CAD build for the part. Positions are in the model's coordinates, mm. A direction names the side the tool comes from. Coordinates: 2 decimals unless noted, no trailing zeros. Order: outer loops, then holes, each group sorted by start corner. A loop starts at its lowest first (then second) coordinate and runs counter-clockwise, first axis right, second up. Notation, with made-up numbers: (52, 51.5) - (61, 51.5) arc R31 cw to (61, 89.5) - close; hole circle Ø6 at (70, 83). An arc over 180 degrees is marked (long way). Write each question's results on one line, items separated by ' | '. Start each with the question number.
Q1. Band-saw the part on D-D, the plane z = 24.4. Write the cut outline in (x, y), then the cut area to 3 significant figures.
Q2. Band-saw the part on B-B, the plane z = -5.5. Write the cut outline in (x, y), then the cut area to 3 significant figures.
Q3. Band-saw the part on C-C, the plane y = 12. Write the cut outline in (x, z).
Q4. Band-saw the part on A-A, the plane x = 5.2. Write the cut outline in (y, z).
Q5. Pin check, flat tips, straight feed: P1, Ø1, axis at x = -9.5, y = 10, coming from the -Z side; P2, Ø3.5, axis at x = 7, y = 16.5, coming from the +Z side; P3, Ø3.5, axis at x = 5.2, z = 23.8, coming from the -Y side. Stop position of each tip, or through.
Q6. Wall check: probe 1 along Z at (x, y) = (5.2, 26.4); probe 2 along X at (y, z) = (26.3, -23.8); probe 3 along Z at (x, y) = (-7, 20.5). Give the ranges that are in metal, low to high.
Q7. Which spindle directions (+Z, -Z, +X, -X, +Y, -Y) get a long thin tool onto all of the face, cutting with end or side? Do faces 4 (the flat face through (-3, 26, -22.5)), 5 (the flat face through (-10.1, 13, -26)), 6 (the flat face through (1, 24.9, 24)). Say none if no direction does.
Q8. Pull direction Z, two halves, no side cores. Call faces 1 (the flat face through (-11, 26.9, 0)), 2 (the flat face through (-11, 18, 27.5)), 3 (the flat face through (0, 14, 20.1)): released by +Z, released by -Z, zero draft, split by the parting line, or undercut.
```python
from build123d import *

# Parameters (mm, degrees)
SKETCH2_W           = 75
SKETCH2_H           = 8
SKETCH2_R           = 1.6
BOSS_EXTRUDE1_DEPTH = 2
SKETCH3_W           = 25
SKETCH3_H           = 18.5
BOSS_EXTRUDE2_DEPTH = 2
SKETCH4_W           = 25
SKETCH4_H           = 2
BOSS_EXTRUDE3_DEPTH = 18.5
SKETCH5_W           = 10.2
SKETCH5_H           = 40.2
CUT_EXTRUDE1_DEPTH  = 18.5
SKETCH6_W           = 10.2
SKETCH6_H           = 40.2
BOSS_EXTRUDE4_DEPTH = 24.9
SKETCH8_W           = 25
SKETCH8_H           = 7
BOSS_EXTRUDE5_DEPTH = 2
SKETCH9_R           = 1.6
CUT_EXTRUDE2_DEPTH  = 2
SKETCH10_W          = 20.2
SKETCH10_H          = 40.2
CUT_EXTRUDE3_DEPTH  = 77
SKETCH11_W          = 7
SKETCH11_H          = 2.4
CUT_EXTRUDE4_DEPTH  = 77
SKETCH12_W          = 2.4
SKETCH12_H          = 7
BOSS_EXTRUDE6_DEPTH = 24.9
SKETCH13_W          = 4
SKETCH13_H          = 4
CUT_EXTRUDE5_DEPTH  = 77
SKETCH14_W          = 25
SKETCH14_H          = 8
SKETCH14_R          = 1.6
BOSS_EXTRUDE7_DEPTH = 2
CUT_EXTRUDE6_DEPTH  = 2
CHAMFER1_SIZE       = 10
CUT_EXTRUDE7_DEPTH  = 1.2
SKETCH17_W          = 20.2
SKETCH17_H          = 22.9
CUT_EXTRUDE8_DEPTH  = 1.2
CUT_EXTRUDE9_DEPTH  = 2
CUT_EXTRUDE10_DEPTH = 2
SKETCH20_W          = 25
SKETCH20_H          = 8
CUT_EXTRUDE11_DEPTH = 156
SKETCH21_W          = 6.2
SKETCH21_H          = 22.9
CUT_EXTRUDE12_DEPTH = 55
SKETCH22_R          = 1.6
CUT_EXTRUDE13_DEPTH = 55


with BuildPart() as part:
    # Sketch2 → Boss-Extrude1 (new body)
    with BuildSketch(Plane(origin=(0, 0, 0), x_dir=(1, 0, 0), z_dir=(0, 1, 0))):
        Rectangle(SKETCH2_W, SKETCH2_H)
        with Locations((-31.75, 0)):
            Circle(SKETCH2_R, mode=Mode.SUBTRACT)
        with Locations((31.75, 0)):
            Circle(SKETCH2_R, mode=Mode.SUBTRACT)
    extrude(amount=BOSS_EXTRUDE1_DEPTH)

    # Sketch3 → Boss-Extrude2 (add)
    with BuildSketch(Plane(origin=(0, 2, 0), x_dir=(1, 0, 0), z_dir=(0, 1, 0))):
        with Locations((0, -13.25)):
            Rectangle(SKETCH3_W, SKETCH3_H)
    extrude(amount=-BOSS_EXTRUDE2_DEPTH)

    # Sketch4 → Boss-Extrude3 (add)
    with BuildSketch(Plane(origin=(0, 0, -4), x_dir=(-1, 0, 0), z_dir=(0, 0, -1))):
        with Locations((0, 1)):
            Rectangle(SKETCH4_W, SKETCH4_H)
    extrude(amount=BOSS_EXTRUDE3_DEPTH)

    # Sketch5 → Cut-Extrude1 (cut)
    with BuildSketch(Plane(origin=(0, 2, 0), x_dir=(1, 0, 0), z_dir=(0, 1, 0))):
        Rectangle(SKETCH5_W, SKETCH5_H)
    extrude(amount=-CUT_EXTRUDE1_DEPTH, mode=Mode.SUBTRACT)

    # Sketch6 → Boss-Extrude4 (add)
    with BuildSketch(Plane(origin=(0, 2, 0), x_dir=(1, 0, 0), z_dir=(0, 1, 0))):
        Polygon((-12.5, 4), (-12.5, -4), (-12.5, -22.5), (12.5, -22.5), (12.5, -4), (12.5, 4), (12.5, 22.5), (-12.5, 22.5), align=None)
        Rectangle(SKETCH6_W, SKETCH6_H, mode=Mode.SUBTRACT)
    extrude(amount=BOSS_EXTRUDE4_DEPTH)

    # Sketch8 → Boss-Extrude5 (add)
    with BuildSketch(Plane(origin=(0, 26.9, 0), x_dir=(1, 0, 0), z_dir=(0, 1, 0))):
        with Locations((0, 26)):
            Rectangle(SKETCH8_W, SKETCH8_H)
        with Locations((0, -26)):
            Rectangle(SKETCH8_W, SKETCH8_H)
    extrude(amount=-BOSS_EXTRUDE5_DEPTH)

    # Sketch9 → Cut-Extrude2 (cut)
    with BuildSketch(Plane.XZ.offset(-24.9)):
        with Locations((5.2, 23.8)):
            Circle(SKETCH9_R)
        with Locations((-5.2, 23.8)):
            Circle(SKETCH9_R)
        with Locations((-5.2, -23.8)):
            Circle(SKETCH9_R)
        with Locations((5.2, -23.8)):
            Circle(SKETCH9_R)
    extrude(amount=-CUT_EXTRUDE2_DEPTH, mode=Mode.SUBTRACT)

    # Sketch10 → Cut-Extrude3 (cut)
    with BuildSketch(Plane.XZ):
        Rectangle(SKETCH10_W, SKETCH10_H)
    extrude(amount=-CUT_EXTRUDE3_DEPTH, mode=Mode.SUBTRACT)

    # Sketch11 → Cut-Extrude4 (cut)
    with BuildSketch(Plane.XZ):
        with Locations((0, -21.3)):
            Rectangle(SKETCH11_W, SKETCH11_H)
    extrude(amount=-CUT_EXTRUDE4_DEPTH, mode=Mode.SUBTRACT)

    # Sketch12 → Boss-Extrude6 (add)
    with BuildSketch(Plane.XZ):
        with Locations((-11.3, 26)):
            Rectangle(SKETCH12_W, SKETCH12_H)
        with Locations((-11.3, -26)):
            Rectangle(SKETCH12_W, SKETCH12_H)
        with Locations((11.3, 26)):
            Rectangle(SKETCH12_W, SKETCH12_H)
        with Locations((11.3, -26)):
            Rectangle(SKETCH12_W, SKETCH12_H)
    extrude(amount=-BOSS_EXTRUDE6_DEPTH)

    # Sketch13 → Cut-Extrude5 (cut)
    with BuildSketch(Plane(origin=(0, 26.9, 0), x_dir=(1, 0, 0), z_dir=(0, 1, 0))):
        with Locations((0, 22.5)):
            Rectangle(SKETCH13_W, SKETCH13_H)
    extrude(amount=-CUT_EXTRUDE5_DEPTH, mode=Mode.SUBTRACT)

    # Sketch14 → Boss-Extrude7 (add)
    with BuildSketch(Plane(origin=(0, 2, 0), x_dir=(1, 0, 0), z_dir=(0, 1, 0))):
        with Locations((-25, 0)):
            Rectangle(SKETCH14_W, SKETCH14_H)
        with Locations((-31.75, 0)):
            Circle(SKETCH14_R, mode=Mode.SUBTRACT)
        with Locations((25, 0)):
            Rectangle(SKETCH14_W, SKETCH14_H)
        with Locations((31.75, 0)):
            Circle(SKETCH14_R, mode=Mode.SUBTRACT)
    extrude(amount=BOSS_EXTRUDE7_DEPTH)

    # Sketch15 → Cut-Extrude6 (cut)
    with BuildSketch(Plane.XZ):
        Polygon((10.1, -20.1), (3.5, -20.1), (3.5, -22.5), (10.1, -22.5), (10.1, -29.5), (12.5, -29.5), (12.5, -4), (37.5, -4), (37.5, 4), (12.5, 4), (12.5, 29.5), (10.1, 29.5), (10.1, 22.5), (-10.1, 22.5), (-10.1, 29.5), (-12.5, 29.5), (-12.5, 4), (-37.5, 4), (-37.5, -4), (-12.5, -4), (-12.5, -29.5), (-10.1, -29.5), (-10.1, -22.5), (-3.5, -22.5), (-3.5, -20.1), (-10.1, -20.1), (-10.1, 20.1), (10.1, 20.1), align=None)
    extrude(amount=-CUT_EXTRUDE6_DEPTH, mode=Mode.SUBTRACT)

    # Chamfer1
    chamfer1_edges = [part.edges().sort_by_distance(p)[0] for p in [
        (-12.5, 4, 0),
        (12.5, 4, 0),
    ]]
    chamfer(chamfer1_edges, length=CHAMFER1_SIZE)

    # Sketch16 → Cut-Extrude7 (cut)
    with BuildSketch(Plane.XY.offset(22.5)):
        Polygon((-10.1, 2), (10.1, 2), (10.1, 24.9), (6.132737905, 24.9), (4.267262095, 24.9), (-4.267262095, 24.9), (-6.132737905, 24.9), (-10.1, 24.9), align=None)
    extrude(amount=-CUT_EXTRUDE7_DEPTH, mode=Mode.SUBTRACT)

    # Sketch17 → Cut-Extrude8 (cut)
    with BuildSketch(Plane(origin=(0, 0, -22.5), x_dir=(-1, 0, 0), z_dir=(0, 0, -1))):
        with Locations((0, 13.45)):
            Rectangle(SKETCH17_W, SKETCH17_H)
    extrude(amount=-CUT_EXTRUDE8_DEPTH, mode=Mode.SUBTRACT)

    # Sketch18 → Cut-Extrude9 (cut)
    with BuildSketch(Plane(origin=(0, 0, -29.5), x_dir=(-1, 0, 0), z_dir=(0, 0, -1))):
        Polygon((10.1, 2), (12.5, 2), (12.5, 26.9), (-12.5, 26.9), (-12.5, 2), (-10.1, 2), (-10.1, 24.9), (10.1, 24.9), align=None)
    extrude(amount=-CUT_EXTRUDE9_DEPTH, mode=Mode.SUBTRACT)

    # Sketch19 → Cut-Extrude10 (cut)
    with BuildSketch(Plane.XY.offset(29.5)):
        Polygon((10.1, 2), (12.5, 2), (12.5, 26.9), (-12.5, 26.9), (-12.5, 2), (-10.1, 2), (-10.1, 24.9), (10.1, 24.9), align=None)
    extrude(amount=-CUT_EXTRUDE10_DEPTH, mode=Mode.SUBTRACT)

    # Sketch20 → Cut-Extrude11 (cut)
    with BuildSketch(Plane.XZ.offset(-2)):
        with Locations((-25, 0)):
            Rectangle(SKETCH20_W, SKETCH20_H)
        with Locations((25, 0)):
            Rectangle(SKETCH20_W, SKETCH20_H)
    extrude(amount=-CUT_EXTRUDE11_DEPTH, mode=Mode.SUBTRACT)

    # Sketch21 → Cut-Extrude12 (cut)
    with BuildSketch(Plane(origin=(-10.1, 0, 0), x_dir=(0, 0, -1), z_dir=(1, 0, 0))):
        with Locations((-24.4, 13.45)):
            Rectangle(SKETCH21_W, SKETCH21_H)
        with Locations((24.4, 13.45)):
            Rectangle(SKETCH21_W, SKETCH21_H)
    extrude(amount=CUT_EXTRUDE12_DEPTH, mode=Mode.SUBTRACT)

    # Sketch22 → Cut-Extrude13 (cut)
    with BuildSketch(Plane(origin=(-10.1, 0, 0), x_dir=(0, 0, -1), z_dir=(1, 0, 0))):
        with Locations((-24.4, 12)):
            Circle(SKETCH22_R)
        with Locations((24.4, 12)):
            Circle(SKETCH22_R)
    extrude(amount=-CUT_EXTRUDE13_DEPTH, mode=Mode.SUBTRACT)


solid = part.part
```
Results below:
1) outline: (-12.5, 2) - (-10.1, 2) - (-10.1, 10.4) - (-12.5, 10.4) - close; (-12.5, 13.6) - (-10.1, 13.6) - (-10.1, 24.9) - (-6.68, 24.9) - (-6.68, 26.9) - (-12.5, 26.9) - close; (-3.72, 24.9) - (3.72, 24.9) - (3.72, 26.9) - (-3.72, 26.9) - close; (6.68, 24.9) - (12.5, 24.9) - (12.5, 26.9) - (6.68, 26.9) - close | area: 85.4 mm²
2) outline: (-12.5, 2) - (-10.1, 2) - (-10.1, 26.9) - (-12.5, 26.9) - close; (10.1, 2) - (12.5, 2) - (12.5, 26.9) - (10.1, 26.9) - close | area: 120 mm²
3) outline: (-12.5, -27.5) - (-10.1, -27.5) - (-10.1, -26) - (-12.5, -26) - close; (-12.5, -22.8) - (-10.1, -22.8) - (-10.1, -21.3) - (-3.5, -21.3) - (-3.5, -20.1) - (-10.1, -20.1) - (-10.1, 20.1) - (10.1, 20.1) - (10.1, -20.1) - (3.5, -20.1) - (3.5, -21.3) - (12.5, -21.3) - (12.5, 21.3) - (-10.1, 21.3) - (-10.1, 22.8) - (-12.5, 22.8) - close; (-12.5, 26) - (-10.1, 26) - (-10.1, 27.5) - (-12.5, 27.5) - close
4) outline: (2, -21.3) - (24.9, -21.3) - (24.9, -22.2) - (26.9, -22.2) - (26.9, -20.1) - (2, -20.1) - close; (2, 20.1) - (26.9, 20.1) - (26.9, 22.2) - (24.9, 22.2) - (24.9, 21.3) - (2, 21.3) - close; (24.9, -27.5) - (26.9, -27.5) - (26.9, -25.4) - (24.9, -25.4) - close; (24.9, 25.4) - (26.9, 25.4) - (26.9, 27.5) - (24.9, 27.5) - close
5) P1: stops at z = -21.3 | P2: stops at z = 21.3 | P3: stops at y = 24.9
6) probe 1: z = -27.5 to -25.4, -22.2 to -20.1, 20.1 to 22.2, 25.4 to 27.5 | probe 2: x = -12.5 to -6.8, -3.6 to -2, 2 to 3.6, 6.8 to 12.5 | probe 3: z = -21.3 to -20.1, 20.1 to 21.3
7) face 4: +Y, -Y | face 5: -Z, +X, -Y | face 6: +Z, +X, -Y
8) face 1: zero draft | face 2: released by +Z | face 3: undercut
